Check sheet for the modelled part. Datum: model origin and axes. Units: mm. A direction names the side the tool comes from. Coordinates: 2 decimals unless noted, no trailing zeros. Write each loop counter-clockwise with the first axis right and the second up, starting at its lowest first coordinate (ties: lowest second). Pieces come first, ordered by that corner, then holes. Notation, with made-up numbers: (69, -13) -> (91, -13) arc R30 cw to (91, 25) -> close; hole circle Ø1 at (-40, 43). An arc over 180 degrees is marked (long way). One line per item, written item: value. Start each with the question number.
1) Gauge pin test, flat ends, axial feed: P1, Ø1.5, axis at y = -34.5, z = 27, coming from the +X side; P2, Ø20, axis at x = 27.5, z = -1, coming from the +Y side; P3, Ø4.5, axis at x = -24.5, y = -42.5, coming from the +Z side; P4, Ø1.5, axis at x = 22.5, y = -1.5, coming from the +Z side. Record the tip position at first contact, or that the pin passes through.
2) Sectioned sample at A-A on y = -25. Enter the section's corners in (x, z).
3) Sectioned sample at D-D on y = -12.5. Enter the section's corners in (x, z).
4) Draft check along X on faces 5 (the flat face through (-38, -42, 0)), 6 (the cylindrical face through (-29.16, -42.03, 1.05)), 7 (the flat face through (0, -19, -35)). Enter one of: +X half, -X half, draft (parallel to the pull), parting line (faces both ways), or undercut.
5) Scan lines: line 1 along Y through (x, z) = (0, 31.5); line 2 along Z through (x, y) = (14, 2); line 3 along Y through (x, z) = (-20.5, 10). Record each from-to range of solid material in increasing order. Write a range as [from, to].
6) Sectioned sample at B-B on z = 0. Enter the section's corners in (x, y).
7) Set-up check for faces 1 (the flat face through (29, -42, -25)), 2 (the flat face through (-29, -42, 25)), 3 (the flat face through (0, -28, 0)), 4 (the flat face through (-13.3, 4.9, 25)): record each of +Z, -Z, +X, -X, +Y, -Y from which the full face is reachable in a straight line by a thin tool's end or side.
8) Sectioned sample at C-C on x = -32.5. Enter the section's corners in (y, z).
```python
from build123d import *

# Parameters (mm, degrees)
SKETCH002_AS_DRAWN_W                 = 76
SKETCH002_AS_DRAWN_H                 = 50
SKETCH002_AS_DRAWN_R                 = 3.5
EXTRUDE003_DEPTH                     = 4
EXTRUDE003_ONTO_SKETCH002_ROLL_ANGLE = 90
CYLINDER_R                           = 16.25
CYLINDER_DEPTH                       = 10
SKETCH_R                             = 14
EXTRUDE001_DEPTH                     = 12
CYLINDER001_R                        = 16.25
CYLINDER001_DEPTH                    = 10
EXTRUDE_DEPTH                        = 12
SKETCH001_AS_DRAWN_W                 = 40
SKETCH001_AS_DRAWN_H                 = 70
EXTRUDE002_DEPTH                     = 16
EXTRUDE002_ONTO_SKETCH001_ROLL_ANGLE = 90


with BuildPart() as extrude003:
    # Sketch002 as drawn → Extrude003 (new)
    with BuildSketch(Plane.XY):
        Rectangle(SKETCH002_AS_DRAWN_W, SKETCH002_AS_DRAWN_H)
        with Locations((-32.5, 0)):
            Circle(SKETCH002_AS_DRAWN_R, mode=Mode.SUBTRACT)
        with Locations((32.5, 0)):
            Circle(SKETCH002_AS_DRAWN_R, mode=Mode.SUBTRACT)
    extrude(amount=-EXTRUDE003_DEPTH)


with BuildPart() as extrude003_1:
    # Extrude003 onto Sketch002 roll: moved
    add(extrude003.part.rotate(Axis((0, 0, 0), (1, 0, 0)), EXTRUDE003_ONTO_SKETCH002_ROLL_ANGLE))


with BuildPart() as extrude003_2:
    # Extrude003 onto Sketch002 placement: moved
    add(extrude003_1.part)


with BuildPart() as extrude003_3:
    # Extrude003 placement: moved
    add(extrude003_2.part.moved(Location((0, -44, 0))))


with BuildPart() as cylinder:
    # Cylinder → Cylinder (new body)
    with BuildSketch(Plane.XY):
        Circle(CYLINDER_R)
    extrude(amount=CYLINDER_DEPTH)


with BuildPart() as obj1:
    # Sketch → Extrude001 (new body)
    with BuildSketch(Plane.XY):
        with BuildLine():
            ThreePointArc((20, 0), (0, 20), (-20, 0))
            Line((-20, 0), (-20, -40))
            Line((-20, -40), (20, -40))
            Line((20, -40), (20, 0))
        make_face()
        Circle(SKETCH_R, mode=Mode.SUBTRACT)
    extrude(amount=EXTRUDE001_DEPTH)

    # Cut: cut Cylinder
    add(cylinder.part, mode=Mode.SUBTRACT)


with BuildPart() as obj1_1:
    # Cut placement: moved
    add(obj1.part.moved(Location((0, 0, -35))))


with BuildPart() as cylinder001:
    # Cylinder001 → Cylinder001 (new body)
    with BuildSketch(Plane.XY.offset(2)):
        Circle(CYLINDER001_R)
    extrude(amount=CYLINDER001_DEPTH)


with BuildPart() as bearing_nest_r_cut:
    # Sketch → Extrude (new body)
    with BuildSketch(Plane.XY):
        with BuildLine():
            ThreePointArc((20, 0), (0, 20), (-20, 0))
            Line((-20, 0), (-20, -40))
            Line((-20, -40), (20, -40))
            Line((20, -40), (20, 0))
        make_face()
        Circle(SKETCH_R, mode=Mode.SUBTRACT)
    extrude(amount=EXTRUDE_DEPTH)

    # Cut001: cut Cylinder001
    add(cylinder001.part, mode=Mode.SUBTRACT)


with BuildPart() as bearing_nest_r_cut_1:
    # Cut001 placement: moved
    add(bearing_nest_r_cut.part.moved(Location((0, 0, 23))))


with BuildPart() as fusion:
    # Sketch001 as drawn → Extrude002 (new)
    with BuildSketch(Plane.XY):
        Rectangle(SKETCH001_AS_DRAWN_W, SKETCH001_AS_DRAWN_H)
    extrude(amount=-EXTRUDE002_DEPTH)


with BuildPart() as fusion_1:
    # Extrude002 onto Sketch001 roll: moved
    add(fusion.part.rotate(Axis((0, 0, 0), (1, 0, 0)), EXTRUDE002_ONTO_SKETCH001_ROLL_ANGLE))


with BuildPart() as fusion_2:
    # Extrude002 onto Sketch001 placement: moved
    add(fusion_1.part)


with BuildPart() as fusion_3:
    # Extrude002 placement: moved
    add(fusion_2.part.moved(Location((0, -44, 0))))

    # Fusion: union Extrude003, obj1, bearing-nest-r-cut
    add(extrude003_3.part)
    add(obj1_1.part)
    add(bearing_nest_r_cut_1.part)


solid = fusion_3.part
```
Answers:
1. P1: stops at x = 20
1. P2: stops at y = -28
1. P3: stops at z = 25
1. P4: passes through
2. outline: (-20, -35) -> (20, -35) -> (20, -23) -> (-20, -23) -> close; (-20, 23) -> (20, 23) -> (20, 35) -> (-20, 35) -> close
3. outline: (-20, -35) -> (-10.38, -35) -> (-10.38, -25) -> (-6.3, -25) -> (-6.3, -23) -> (-20, -23) -> close; (-20, 23) -> (-6.3, 23) -> (-6.3, 25) -> (-10.38, 25) -> (-10.38, 35) -> (-20, 35) -> close; (6.3, -25) -> (10.38, -25) -> (10.38, -35) -> (20, -35) -> (20, -23) -> (6.3, -23) -> close; (6.3, 23) -> (20, 23) -> (20, 35) -> (10.38, 35) -> (10.38, 25) -> (6.3, 25) -> close
4. face 5: -X half
4. face 6: undercut
4. face 7: draft
5. line 1: y = [-44, -16.25], [16.25, 20]
5. line 2: z = [-25, -23], [23, 25]
5. line 3: y = [-44, -40]
6. outline: (-38, -44) -> (-36, -44) -> (-36, -40) -> (-38, -40) -> close; (-29, -44) -> (29, -44) -> (29, -40) -> (20, -40) -> (20, -28) -> (-20, -28) -> (-20, -40) -> (-29, -40) -> close; (36, -44) -> (38, -44) -> (38, -40) -> (36, -40) -> close
7. face 1: -Z, +X, +Y, -Y
7. face 2: +Z, -X, +Y, -Y
7. face 3: +X, -X, +Y
7. face 4: +Z
8. outline: (-44, -25) -> (-40, -25) -> (-40, -3.5) -> (-44, -3.5) -> close; (-44, 3.5) -> (-40, 3.5) -> (-40, 25) -> (-44, 25) -> close
